Build history of the part. All positions in model axes, mm. A direction names the side the tool comes from. Give positions to 0.01 mm unless a question says otherwise; leave off trailing zeros. Order: outer loops, then holes, each group sorted by start corner. A loop starts at its lowest first (then second) coordinate and runs counter-clockwise, first axis right, second up. Notation, with made-up numbers: (9.5, 28) - (67.5, 28) arc R33 cw to (67.5, 66) - close; hole circle Ø1 at (26.5, -14). An arc over 180 degrees is marked (long way). Answer in a Markdown table with one row per item.
Autodesk Fusion 360 part; units mm, degrees
sketch "Sketch1" plane through (0, 0, 0) normal (0, 0, 1) x (1, 0, 0)
  line L0 (-25, 50) -> (75, 50)
  line L1 (75, 50) -> (75, -20)
  line L2 (75, -20) -> (-25, -20)
  line L3 (-25, -20) -> (-25, 50)
  dimension "d1" = 100
  dimension "d2" = 70
extrude "Extrude1" add sketch "Sketch1" along normal blind 10
sketch "Sketch2" plane through (0, 0, 0) normal (1, 0, 0) x (0, 1, 0)
  line L0 (-20, 50) -> (-20, -25) construction
  line L1 (50, 50) -> (50, -25) construction
  line L2 (-25, 0) -> (55, 0) construction
  line L3 (15, 50) -> (15, -25) construction
  line L4 (-25, 30) -> (55, 30) construction
  circle A0 centre (15, 30) radius 3
  circle A1 centre (15, 30) radius 30
  circle A2 centre (0, 15) radius 2
  circle A3 centre (15, 30) radius 3
  circle A4 centre (0, 45) radius 2
  circle A5 centre (30, 45) radius 2
  circle A6 centre (15, 30) radius 3
  circle A7 centre (30, 15) radius 2
  circle A8 centre (15, 30) radius 3
  line L5 (59.9207, 15) -> (-20, 15) construction
  line L6 (30, 60) -> (30, -2) construction
  line L7 (0, 60) -> (0, -2) construction
  point P0 (0, 45)
  dimension "d5" = 35
  dimension "d6" = 30
  dimension "d7" = 6
  dimension "d8" = 60
  dimension "d9" = 4
  dimension "d10" = 4
  dimension "d18" = 15
  dimension "d19" = 15
extrude "Extrude2" add sketch "Sketch2" along normal blind 10 from surface at -25 contours A1 | A2 | A4 | A5 | A7
sketch "Sketch3" plane through (0, 0, 0) normal (0, 1, 0) x (1, 0, 0)
  line L0 (-30, 0) -> (80, 0) construction
  line L1 (25, -65) -> (25, 5) construction
  line L2 (-30, -30) -> (80, -30) construction
  line L3 (-25, -65) -> (-25, 5) construction
  line L4 (-35, -15) -> (111.1834, -15) construction
  line L5 (55, -65) -> (55, 5) construction
  line L6 (70, -70) -> (70, 15) construction
  circle A0 centre (55, -30) radius 30
  circle A1 centre (40, -45) radius 2
  circle A2 centre (55, -30) radius 3
  circle A3 centre (70, -45) radius 2
  circle A4 centre (40, -15) radius 2
  circle A5 centre (70, -15) radius 2
  point P0 (70, -15)
  dimension "d14" = 50
  dimension "d15" = 30
  dimension "d20" = 15
  dimension "d21" = 15
  dimension "d53" = 4
extrude "Extrude3" add sketch "Sketch3" against normal blind 10 from surface at 50 contours A0 | A1 | A3 | A4 | A5
ref_plane "WorkPlane1" through (0, -30, 0) normal (0, 1, 0) x (0, 0, 1)
sketch "Sketch4" plane through (0, -30, 0) normal (0, 1, 0) x (1, 0, 0)
  line L0 (85, 0) -> (-35, 0) construction
  line L1 (-35, -7.64) -> (92.4851, -7.64) construction
  line L2 (55, -30) -> (55, 12) construction
  line L3 (25, -75) -> (25, 12.7577) construction
  line L4 (75.0008, -7.64) -> (75.0008, 2)
  circle A0 centre (55, -30) radius 30
  line L5 (88, 0) -> (48, 0)
extrude "Extrude6" cut sketch "Sketch4" against normal blind 10 from surface at 80 contours L4 A0 L5
extrude "Extrude8" cut sketch "Sketch2" against normal blind 8 from surface at -15 contours A2 | A4 | A5 | A7
extrude "Extrude9" cut sketch "Sketch3" along normal blind 8 from surface at 40 contours A1 | A3 | A4 | A5
1. Two-plate mould, pull along Y, no slides. Class faces 1 (the face through (41, 50, 23)), 2 (the face through (-23, 30, 15)), 3 (the face through (75, 10, 5)): +Y half, -Y half, draft (parallel to the pull), parting line (faces both ways), or undercut.
Check result:
| item | result |
|---|---|
| face 1 | +Y half |
| face 2 | undercut |
| face 3 | draft |
2. Cut at C-C on y = 30. Write the cut outline in (x, z), and give its area (3 significant figures).
Check result:
| item | result |
|---|---|
| outline | (-25, 0) - (75, 0) - (75, 10) - (-15, 10) - (-15, 13) - (-23, 13) - (-23, 17) - (-15, 17) - (-15, 43) - (-23, 43) - (-23, 47) - (-15, 47) - (-15, 55.98) - (-25, 55.98) - close |
| area | 1,400 mm² |
3. Drop flat-ended pins along their axis: P1, Ø3, axis at x = 73, y = 37, coming from the +Z side; P2, Ø5, axis at x = 34.5, y = -12, coming from the -Z side; P3, Ø1.2, axis at y = 29.5, z = 15, coming from the +X side; P4, Ø2.5, axis at x = 40, z = 15, coming from the -Y side. Give the stop position or say it passes through.
Check result:
| item | result |
|---|---|
| P1 | stops at z = 10 |
| P2 | stops at z = 0 |
| P3 | stops at x = -23 |
| P4 | stops at y = 48 |
4. Probe line 1 (X direction, y = 43.25, z = 30); line 2 (Z direction, x = -18, y = 15); line 3 (Z direction, x = 40, y = 45.75). List the from-to ranges inside material, lowest first.
Check result:
| item | result |
|---|---|
| line 1 | x = -25 to -15, 25 to 52, 58 to 85 |
| line 2 | z = 0 to 27, 33 to 60 |
| line 3 | z = 0 to 13, 17 to 43, 47 to 55.98 |
5. Cut at A-A on z = 45. Write the cut outline in (x, y).
Check result:
| item | result |
|---|---|
| outline | (-25, -10.98) - (-15, -10.98) - (-15, -2) - (-23, -2) - (-23, 2) - (-15, 2) - (-15, 28) - (-23, 28) - (-23, 32) - (-15, 32) - (-15, 40.98) - (-25, 40.98) - close; (29.02, 40) - (38, 40) - (38, 48) - (42, 48) - (42, 40) - (68, 40) - (68, 48) - (72, 48) - (72, 40) - (80.98, 40) - (80.98, 50) - (29.02, 50) - close |
6. Cut at B-B on x = 62.5. Write the cut outline in (y, z), and give its area (3 significant figures).
Check result:
| item | result |
|---|---|
| outline | (-20, 0) - (40, 0) - (40, 0.95) - (50, 0.95) - (50, 59.05) - (40, 59.05) - (40, 10) - (-20, 10) - close |
| area | 1,180 mm² |
7. Which spindle directions (+Z, -Z, +X, -X, +Y, -Y) get a long thin tool onto all of the face, cutting with end or side? Do faces 4 (the face through (-18.944, 0.923, 43.226)), 5 (the face through (40, 48, 15)), 6 (the face through (70, 40, 2)), 7 (the face through (26, -20, 5)). Say none if no direction does.
Check result:
| item | result |
|---|---|
| face 4 | +X |
| face 5 | -Y |
| face 6 | -Z, +X, +Y |
| face 7 | +Z, -Z, +X, -X, -Y |
8. Cut at D-D on x = 48. Write the cut outline in (y, z), and give its area (3 significant figures).
Check result:
| item | result |
|---|---|
| outline | (-20, 0) - (50, 0) - (50, 59.17) - (40, 59.17) - (40, 10) - (-20, 10) - close |
| area | 1,190 mm² |
